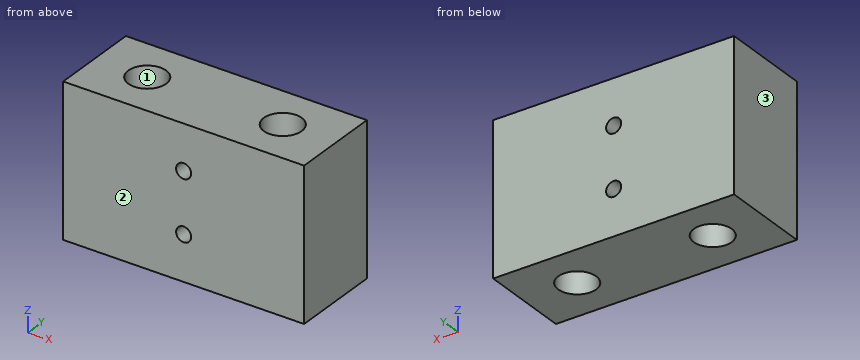
from build123d import *

# Parameters (mm, degrees)
SKETCH1_W           = 50.8
SKETCH1_H           = 19.05
SKETCH1_R           = 4
BOSS_EXTRUDE1_DEPTH = 31.75
SKETCH2_R           = 1.5875
CUT_EXTRUDE1_DEPTH  = 45.901280605


with BuildPart() as part:
    # Sketch1 → Boss-Extrude1 (new body)
    with BuildSketch(Plane.XY):
        Rectangle(SKETCH1_W, SKETCH1_H)
        with Locations((-14.2875, 0)):
            Circle(SKETCH1_R, mode=Mode.SUBTRACT)
        with Locations((14.2875, 0)):
            Circle(SKETCH1_R, mode=Mode.SUBTRACT)
    extrude(amount=BOSS_EXTRUDE1_DEPTH)

    # Sketch2 → Cut-Extrude1 (cut, through all)
    with BuildSketch(Plane(origin=(0, 9.525, 0), x_dir=(1, 0, 0), z_dir=(0, 1, 0))):
        with Locations(Location((0, -9.525, 0), (0, 0, 270))):
            Circle(SKETCH2_R)
        with Locations(Location((0, -22.225, 0), (0, 0, 270))):
            Circle(SKETCH2_R)
    extrude(amount=-CUT_EXTRUDE1_DEPTH, mode=Mode.SUBTRACT)


solid = part.part
Input: part model. Units: mm. Frame: model coordinates. Face numbers are marked on the shaded views. Coordinates: 2 decimals unless noted, no trailing zeros. Loops run counter-clockwise (first coordinate to the right, second up) from the corner with the lowest first, then second, coordinate; pieces in that order, holes last. Notation, with made-up numbers: (58, 88.25) -> (69, 88.25) arc R18 ccw to (69, 108.25) -> close; hole circle Ø11 at (71, -11). An arc over 180 degrees is marked (long way). Write item = value, one per line. Start each with the question number.
Item 1: Cut plane C-C, the plane z = 9. Return loops of the section in (x, y) (1 decimal).
Item 2: Material intervals for line 1 (X direction, y = -2, z = 25); line 2 (X direction, y = -1.75, z = 24.5); line 3 (Y direction, x = 17, z = 5) (3 decimals), sorted ascending.
Item 3: Cut plane A-A, the plane y = 0. Count the separate pieces of the cut face and the enclosed holes in it, plus the area to 3 significant figures.
Item 4: Mould query, pull axis Y, two halves, no side actions, for the marked faces 1, 2 and 3. Classes: pulls with the +Y half, pulls with the -Y half, needs draft (parallel to the pull), parting line crosses it, or undercut.
Item 5: Cut plane D-D, the plane z = 23. Return loops of the section in (x, y) (1 decimal), plus the area to 3 significant figures.
Ans:
q1.outline = (-25.4, -9.5) -> (-1.5, -9.5) -> (-1.5, 9.5) -> (-25.4, 9.5) -> close; (1.5, -9.5) -> (25.4, -9.5) -> (25.4, 9.5) -> (1.5, 9.5) -> close; hole circle Ø8 at (-14.3, 0); hole circle Ø8 at (14.3, 0)
q2.line_1 = -25.4 to -17.75, -10.82 to 10.82, 17.75 to 25.4
q2.line_2 = -25.4 to -17.88, -10.69 to 10.69, 17.88 to 25.4
q2.line_3 = -9.525 to -2.94, 2.94 to 9.525
q3.separate_pieces = 3
q3.enclosed_holes = 2
q3.area = 1,090 mm²
q4.face_1 = undercut
q4.face_2 = pulls with the -Y half
q4.face_3 = needs draft
q5.outline = (-25.4, -9.5) -> (-1.4, -9.5) -> (-1.4, 9.5) -> (-25.4, 9.5) -> close; (1.4, -9.5) -> (25.4, -9.5) -> (25.4, 9.5) -> (1.4, 9.5) -> close; hole circle Ø8 at (-14.3, 0); hole circle Ø8 at (14.3, 0)
q5.area = 814 mm²
